from build123d import *

# Parameters (mm, degrees)
SKETCH1_R                               = 55
BOSS_EXTRUDE1_DEPTH                     = 20
SKETCH2_R                               = 27.5
BOSS_EXTRUDE2_DEPTH                     = 10
SKETCH6_R                               = 23.5
CUT_EXTRUDE1_DEPTH                      = 15
FILLET1_R                               = 5
CBORE_FOR_M8_HEX_HEAD_BOLT1_D           = 9
CBORE_FOR_M8_HEX_HEAD_BOLT1_CBORE_D     = 18.011
CBORE_FOR_M8_HEX_HEAD_BOLT1_CBORE_DEPTH = 5.3
FILLET2_R                               = 4


with BuildPart() as part:
    # Sketch1 → Boss-Extrude1 (new body)
    with BuildSketch(Plane(origin=(0, 0, 0), x_dir=(1, 0, 0), z_dir=(0, 1, 0))):
        with Locations(Location((0, 0, 0), (0, 0, 270))):
            Circle(SKETCH1_R)
    extrude(amount=BOSS_EXTRUDE1_DEPTH)

    # Sketch2 → Boss-Extrude2 (add)
    with BuildSketch(Plane(origin=(0, 20, 0), x_dir=(1, 0, 0), z_dir=(0, 1, 0))):
        with Locations(Location((0, 0, 0), (0, 0, 270))):
            Circle(SKETCH2_R)
    extrude(amount=BOSS_EXTRUDE2_DEPTH)

    # Sketch6 → Cut-Extrude1 (cut)
    with BuildSketch(Plane(origin=(0, 30, 0), x_dir=(1, 0, 0), z_dir=(0, 1, 0))):
        with Locations(Location((0, 0, 0), (0, 0, 270))):
            Circle(SKETCH6_R)
    extrude(amount=-CUT_EXTRUDE1_DEPTH, mode=Mode.SUBTRACT)

    # Fillet1
    fillet1_edges = [part.edges().sort_by_distance(p)[0] for p in [
        (0, 20, -27.5),
    ]]
    fillet(fillet1_edges, radius=FILLET1_R)

    # CBORE for M8 Hex Head Bolt1 (through all)
    with Locations(Plane(origin=(27.5, 0, -27.5), x_dir=(0, 0, -1), z_dir=(0, -1, 0))):
        with Locations((0, 0), (0, -55), (-55, -55), (-55, 0)):
            CounterBoreHole(CBORE_FOR_M8_HEX_HEAD_BOLT1_D / 2, CBORE_FOR_M8_HEX_HEAD_BOLT1_CBORE_D / 2, CBORE_FOR_M8_HEX_HEAD_BOLT1_CBORE_DEPTH)

    # Fillet2
    fillet2_edges = [part.edges().sort_by_distance(p)[0] for p in [
        (0, 0, -55),
    ]]
    fillet(fillet2_edges, radius=FILLET2_R)


solid = part.part
Can you work these out from the model? Positions are in its coordinate system, mm. A direction names the side the tool comes from. Coordinates: 2 decimals unless noted, no trailing zeros. Order: outer loops, then holes, each group sorted by start corner. A loop starts at its lowest first (then second) coordinate and runs counter-clockwise, first axis right, second up. Notation, with made-up numbers: (68, 71) - (93, 71) arc R21 ccw to (93, 96) - close; hole circle Ø8 at (26.5, 9). An arc over 180 degrees is marked (long way). Answer as a JSON object with one key per item and string values. Group by question number.
Q1. On a 3-axis mill with a long thin cutter (end or side, diameter ignored), from which of +Z, -Z, +X, -X, +Y, -Y can I reach the whole of each face in a straight line? I mean faces 1 (the face through (31.294, 12.753, -25.081)), 2 (the face through (-36.29, 2.61, -25.55)), 3 (the face through (-24.397, 27.465, 12.69)). Say none if no direction works.
Q2. Imagine slicing it at D-D (y = 23.5). Please give me the cut outline in (x, z), and give its area (3 significant figures).
Q3. I need wall thicknesses on line 1 (X direction, y = 4.75, z = 31); line 2 (Z direction, x = -31.5, y = 7.5); line 3 (X direction, y = 3.15, z = -27.5). Which ranges of each line are inside material? Lowest first, please. Write a range as from..to.
Q4. Will these pins go through, and if not, where does the flat tip stop? P1, Ø3, axis at y = 23, z = -4.5, coming from the -X side; P2, Ø20, axis at x = 31.5, z = 28.5, coming from the -Y side; P3, Ø3, axis at y = 12, z = -39.5, coming from the -X side; P4, Ø16, axis at x = 27.5, z = 27.5, coming from the +Y side.
Q5. Imagine slicing it at B-B (x = 0). Please give me the cut outline in (y, z), and give its area (3 significant figures).
Q6. We'd pull the mould along Z, two halves only. Please class faces 4 (the face through (-29, 5.3, -23)), 5 (the face through (1, 0, -1)), 6 (the face through (-48.794, 11.888, 25.379)): +Z half, -Z half, draft (parallel to the pull), parting line (faces both ways), or undercut.
Q7. Imagine slicing it at C-C (y = 13.25). Please give me the cut outline in (x, z), and give its area (3 significant figures).
Q8. Imagine slicing it at A-A (z = 0). Please give me the cut outline in (x, y), and give its area (3 significant figures).
Determined:
{
 "1": {"face 1": "+Y, -Y", "face 2": "-Y", "face 3": "+Y"},
 "2": {"outline": "circle Ø55.46 at (0, 0); hole circle Ø47 at (0, 0)", "area": "681 mm2"},
 "3": {"line 1": "x = -45.43..-35.8, -19.2..19.2, 35.8..45.43", "line 2": "z = -45.09..-29.56, -25.44..25.44, 29.56..45.09", "line 3": "x = -47.53..-36.51, -18.49..18.49, 36.51..47.53"},
 "4": {"P1": "stops at x = -28.59", "P2": "stops at y = 0", "P3": "stops at x = -39.76", "P4": "stops at y = 20.27"},
 "5": {"outline": "(0, -51) arc R4 ccw to (4, -55) - (20, -55) - (20, -32.5) arc R5 cw to (25, -27.5) - (30, -27.5) - (30, -23.5) - (15, -23.5) - (15, 23.5) - (30, 23.5) - (30, 27.5) - (25, 27.5) arc R5 cw to (20, 32.5) - (20, 55) - (4, 55) arc R4 ccw to (0, 51) - close", "area": "2,050 mm2"},
 "6": {"face 4": "undercut", "face 5": "draft", "face 6": "parting line"},
 "7": {"outline": "circle Ø110 at (0, 0); hole circle Ø9 at (-27.5, -27.5); hole circle Ø9 at (-27.5, 27.5); hole circle Ø9 at (27.5, -27.5); hole circle Ø9 at (27.5, 27.5)", "area": "9,250 mm2"},
 "8": {"outline": "(-55, 4) arc R4 ccw to (-51, 0) - (51, 0) arc R4 ccw to (55, 4) - (55, 20) - (32.5, 20) arc R5 cw to (27.5, 25) - (27.5, 30) - (23.5, 30) - (23.5, 15) - (-23.5, 15) - (-23.5, 30) - (-27.5, 30) - (-27.5, 25) arc R5 cw to (-32.5, 20) - (-55, 20) - close", "area": "2,050 mm2"}
}
